from build123d import *

# Parameters (mm, degrees)
SKETCH1_W               = 20
SKETCH1_H               = 24
BOSS_EXTRUDE1_DEPTH     = 2.5
SKETCH2_W               = 3.6
SKETCH2_H               = 7.5
BOSS_EXTRUDE2_DEPTH     = 5
MIRROR2_COPY_1_SKETCH_W = 3.6
MIRROR2_COPY_1_SKETCH_H = 7.5
MIRROR2_COPY_1_DEPTH    = 5
FILLET1_R               = 0.2
SCALE1_SCALE            = 0.3


with BuildPart() as part:
    # Sketch1 → Boss-Extrude1 (new body, symmetric)
    with BuildSketch(Plane(origin=(0, 0, 0), x_dir=(1, 0, 0), z_dir=(0, 1, 0))):
        Rectangle(SKETCH1_W, SKETCH1_H)
    extrude(amount=BOSS_EXTRUDE1_DEPTH, both=True)

    # Sketch2 → Boss-Extrude2 (add)
    with BuildSketch(Plane(origin=(0, 2.5, 0), x_dir=(1, 0, 0), z_dir=(0, 1, 0))):
        with Locations((-5.3, -15.75)):
            Rectangle(SKETCH2_W, SKETCH2_H)
    boss_extrude2 = extrude(amount=-BOSS_EXTRUDE2_DEPTH)

    # Mirror1: Boss-Extrude2 across plane
    add(boss_extrude2.mirror(Plane(origin=(0, 0, 0), x_dir=(0, 0, 1), z_dir=(1, 0, 0))))

    # Mirror2: Boss-Extrude2 across plane
    add(boss_extrude2.mirror(Plane.XY))

    # Mirror2 copy 1 sketch → Mirror2 copy 1 (add)
    with BuildSketch(Plane(origin=(0, 2.5, 0), x_dir=(-1, 0, 0), z_dir=(0, 1, 0))):
        with Locations((-5.3, -15.75)):
            Rectangle(MIRROR2_COPY_1_SKETCH_W, MIRROR2_COPY_1_SKETCH_H)
    extrude(amount=-MIRROR2_COPY_1_DEPTH)

    # Fillet1
    fillet1_edges = [part.edges().sort_by_distance(p)[0] for p in [
        (-7.1, -2.5, 15.75),
        (-7.1, 0, 19.5),
        (-3.5, -2.5, 15.75),
        (-5.3, -2.5, 19.5),
        (-3.5, 0, 19.5),
        (-7.1, 2.5, 15.75),
        (-5.3, 2.5, 19.5),
        (-3.5, 2.5, 15.75),
        (7.1, 2.5, 15.75),
        (5.3, 2.5, 19.5),
        (7.1, 0, 19.5),
        (3.5, 2.5, 15.75),
        (3.5, 0, 19.5),
        (7.1, -2.5, 15.75),
        (5.3, -2.5, 19.5),
        (3.5, -2.5, 15.75),
        (-7.1, 2.5, -15.75),
        (-5.3, 2.5, -19.5),
        (-7.1, 0, -19.5),
        (-3.5, 2.5, -15.75),
        (-3.5, 0, -19.5),
        (-7.1, -2.5, -15.75),
        (-5.3, -2.5, -19.5),
        (-3.5, -2.5, -15.75),
        (7.1, -2.5, -15.75),
        (7.1, 0, -19.5),
        (3.5, -2.5, -15.75),
        (5.3, -2.5, -19.5),
        (3.5, 0, -19.5),
        (7.1, 2.5, -15.75),
        (5.3, 2.5, -19.5),
        (3.5, 2.5, -15.75),
    ]]
    fillet(fillet1_edges, radius=FILLET1_R)


with BuildPart() as part_1:
    # Scale1: scaled about (0, 0, 0)
    add(part.part.scale(SCALE1_SCALE))


solid = part_1.part
Input: part model. Units: mm. Frame: model coordinates. A direction names the side the tool comes from. Coordinates: 2 decimals unless noted, no trailing zeros. Order: outer loops, then holes, each group sorted by start corner. A loop starts at its lowest first (then second) coordinate and runs counter-clockwise, first axis right, second up. Notation, with made-up numbers: M 22.25,44.25 L 75.25,44.25 A21 ccw 75.25,54.25 Z; hole C 82,-37.75 d11. An arc over 180 degrees is marked long. Answer in a Markdown table with one row per item.
(1) Access query for faces 1 (the flat face through (2.13, 0, -5)), 2 (the flat face through (-1.05, 0, 5)), 3 (the flat face through (1.05, 0, -5)), 4 (the flat face through (2.13, 0, 5)). Directions: +Z, -Z, +X, -X, +Y, -Y. A direction counts if a zero-diameter tool reaches every point of the face in a straight line with its end or side. Return the directions, or none.
Numbers:
| item | result |
|---|---|
| face 1 | -Z, +X, +Y, -Y |
| face 2 | +Z, +Y, -Y |
| face 3 | -Z, +Y, -Y |
| face 4 | +Z, +X, +Y, -Y |
(2) Draft query along X for faces 5 (the flat face through (-2.13, 0, 5)), 6 (the flat face through (1.6, 0, 5.85)), 7 (the flat face through (0, 0, -3.6)). Return one class per face: pulls with the +X half, pulls with the -X half, needs draft (parallel to the pull), parting line crosses it, or undercut.
Numbers:
| item | result |
|---|---|
| face 5 | pulls with the -X half |
| face 6 | needs draft |
| face 7 | undercut |
(3) Contact query for flat-ended pins moving along their axis: pin 1 Ø0.5 at (x, y) = (-2.5, -0.5) entering from -Z; pin 2 Ø0.7 at (y, z) = (-0.5, -4.5) entering from +X; pin 3 Ø0.7 at (y, z) = (0, 4) entering from -X. Output: stop coordinate, or through.
Numbers:
| item | result |
|---|---|
| pin 1 | stops at z = -3.6 |
| pin 2 | stops at x = 2.13 |
| pin 3 | stops at x = -2.13 |
(4) Section query A-A, the plane z = 5. Output: boundary loops of the cut face in (x, y).
Numbers:
| item | result |
|---|---|
| outline | M -2.13,-0.69 A0.06 ccw -2.07,-0.75 L -1.11,-0.75 A0.06 ccw -1.05,-0.69 L -1.05,0.69 A0.06 ccw -1.11,0.75 L -2.07,0.75 A0.06 ccw -2.13,0.69 Z; M 1.05,-0.69 A0.06 ccw 1.11,-0.75 L 2.07,-0.75 A0.06 ccw 2.13,-0.69 L 2.13,0.69 A0.06 ccw 2.07,0.75 L 1.11,0.75 A0.06 ccw 1.05,0.69 Z |
(5) Material intervals for line 1 (Z direction, x = 0.15, y = -0.6); line 2 (X direction, y = -0.3, z = -5), sorted ascending. Write a range as [from, to].
Numbers:
| item | result |
|---|---|
| line 1 | z = [-3.6, 3.6] |
| line 2 | x = [-2.13, -1.05], [1.05, 2.13] |
(6) Section query B-B, the plane y = 0.2. Output: boundary loops of the cut face in (x, z), plus the area to 3 significant figures.
Numbers:
| item | result |
|---|---|
| outline | M -3,-3.6 L -2.13,-3.6 L -2.13,-5.79 A0.06 ccw -2.07,-5.85 L -1.11,-5.85 A0.06 ccw -1.05,-5.79 L -1.05,-3.6 L 1.05,-3.6 L 1.05,-5.79 A0.06 ccw 1.11,-5.85 L 2.07,-5.85 A0.06 ccw 2.13,-5.79 L 2.13,-3.6 L 3,-3.6 L 3,3.6 L 2.13,3.6 L 2.13,5.79 A0.06 ccw 2.07,5.85 L 1.11,5.85 A0.06 ccw 1.05,5.79 L 1.05,3.6 L -1.05,3.6 L -1.05,5.79 A0.06 ccw -1.11,5.85 L -2.07,5.85 A0.06 ccw -2.13,5.79 L -2.13,3.6 L -3,3.6 Z |
| area | 52.9 mm^2 |
(7) Section query C-C, the plane x = 0.6. Output: boundary loops of the cut face in (y, z), plus the area to 3 significant figures.
Numbers:
| item | result |
|---|---|
| outline | M -0.75,-3.6 L 0.75,-3.6 L 0.75,3.6 L -0.75,3.6 Z |
| area | 10.8 mm^2 |
